```python
from build123d import *

# Parameters (mm, degrees)
SKETCH1_R           = 1.6
SKETCH1_R_2         = 2.5
BOSS_EXTRUDE1_DEPTH = 3


with BuildPart() as part:
    # Sketch1 → Boss-Extrude1 (new body)
    with BuildSketch(Plane.XY):
        with BuildLine():
            Line((168.027079905, 1038.043290918), (213.692404138, 1038.043292418))
            ThreePointArc((213.692404138, 1038.043292418), (215.106618088, 1038.62907792), (215.692405461, 1040.043291095))
            Line((215.692405461, 1040.043291095), (215.692425273, 1068.407217461))
            ThreePointArc((215.692425273, 1068.407217461), (215.037497189, 1069.988356706), (213.456358826, 1070.643286918))
            Line((213.456358826, 1070.643286918), (170.527157049, 1070.643286918))
            Line((170.527157049, 1070.643286918), (170.527154049, 1066.109317918))
            ThreePointArc((170.527154049, 1066.109317918), (170.594141198, 1065.85931758), (170.777154049, 1065.67630462))
            ThreePointArc((170.777154049, 1065.67630462), (170.880709235, 1064.889738733), (170.094142887, 1064.993290414))
            ThreePointArc((170.094142887, 1064.993290414), (169.911130301, 1065.176302052), (169.661131049, 1065.243288918))
            Line((169.661131049, 1065.243288918), (168.027102049, 1065.243288918))
            ThreePointArc((168.027102049, 1065.243288918), (167.673548658, 1065.096842309), (167.527102049, 1064.743288918))
            Line((167.527102049, 1064.743288918), (167.527102049, 1059.743291918))
            ThreePointArc((167.527102049, 1059.743291918), (167.673545881, 1059.389741498), (168.027094, 1059.243292111))
            Line((168.027094, 1059.243292111), (169.661121, 1059.243294985))
            ThreePointArc((169.661121, 1059.243294985), (169.911120776, 1059.310282365), (170.094133317, 1059.493294952))
            ThreePointArc((170.094133317, 1059.493294952), (170.880698604, 1059.596848318), (170.77714747, 1058.810282737))
            ThreePointArc((170.77714747, 1058.810282737), (170.594135891, 1058.627270291), (170.527148933, 1058.37727121))
            Line((170.527148933, 1058.37727121), (170.527145536, 1053.243292145))
            Line((170.527145536, 1053.243292145), (173.327145536, 1053.243292145))
            Line((173.327145536, 1053.243292145), (173.327146479, 1054.668300832))
            Line((173.327146479, 1054.668300832), (177.527142575, 1054.668300832))
            Line((177.527142575, 1054.668300832), (177.527142575, 1053.243290914))
            Line((177.527142575, 1053.243290914), (180.527142575, 1053.243292145))
            Line((180.527142575, 1053.243292145), (180.527142575, 1050.043292145))
            Line((180.527142575, 1050.043292145), (177.527142575, 1050.043292145))
            Line((177.527142575, 1050.043292145), (177.527142575, 1048.768300832))
            Line((177.527142575, 1048.768300832), (173.327142575, 1048.768300832))
            Line((173.327142575, 1048.768300832), (173.327143418, 1050.043292145))
            Line((173.327143418, 1050.043292145), (170.527143418, 1050.043292145))
            Line((170.527143418, 1050.043292145), (170.527140021, 1044.909316322))
            ThreePointArc((170.527140021, 1044.909316322), (170.594127154, 1044.659316277), (170.777139735, 1044.476303455))
            ThreePointArc((170.777139735, 1044.476303455), (170.8806944, 1043.689737499), (170.094128121, 1043.793289701))
            ThreePointArc((170.094128121, 1043.793289701), (169.911115656, 1043.97630146), (169.661116448, 1044.043288491))
            Line((169.661116448, 1044.043288491), (168.027087448, 1044.043289572))
            ThreePointArc((168.027087448, 1044.043289572), (167.673533961, 1043.896843197), (167.527087117, 1043.543289903))
            Line((167.527087117, 1043.543289903), (167.527083809, 1038.543292903))
            ThreePointArc((167.527083809, 1038.543292903), (167.673528336, 1038.189739609), (168.027079905, 1038.043290918))
        make_face()
        with Locations((195.192419253, 1056.643286172)):
            Circle(SKETCH1_R, mode=Mode.SUBTRACT)
        with Locations((205.192419253, 1056.643286172)):
            Circle(SKETCH1_R_2, mode=Mode.SUBTRACT)
    extrude(amount=BOSS_EXTRUDE1_DEPTH)


solid = part.part
```
Can you work these out from the model? Positions are in its coordinate system, mm. A direction names the side the tool comes from. Round coordinates to 2 decimals unless told otherwise and drop trailing zeros. Loops run counter-clockwise (first coordinate to the right, second up) from the corner with the lowest first, then second, coordinate; pieces in that order, holes last. Notation, with made-up numbers: M -4.75,33.5 L 10.25,33.5 A22 ccw 10.25,52.5 Z; hole C -27.75,28.25 d4. An arc over 180 degrees is marked long. Write item = value, one per line. Start each with the question number.
(1) Suppose I cut it at B-B on y = 1067. Write out the boundary of the cut face in (x, z).
(2) I need wall thicknesses on line 1 along X through (y, z) = (1058, 2.2); line 2 along Y through (x, z) = (175.5, 0.6); line 3 along X through (y, z) = (1050, 2.5). Which ranges of each line are inside material? Lowest first, please.
(3) Which directions (+Z, -Z, +X, -X, +Y, -Y) give clear straight access to the entire face, cutting with the end or side of a thin tool? Please do faces 1 (the face through (172, 1053.243, 1)), 2 (the face through (191, 1038.043, 1)), 3 (the face through (175, 1054.668, 1)).
(4) Suppose I cut it at D-D on x = 205.5. Write out the boundary of the cut face in (y, z), plus the area to 3 significant figures.
(5) Suppose I cut it at A-A on x = 176.5. Write out the boundary of the cut face in (y, z).
(6) Suppose I cut it at C-C on z = 1. Give the number of separate pieces and of enclosed holes in the cut face, plus the area to 3 significant figures.
(7) I'm going to push flat-ended pins straight in: P1, Ø1.5, axis at y = 1068, z = 1, coming from the -X side; P2, Ø1.2, axis at x = 170.53, y = 1065.24, coming from the -Z side. Where does each tip first touch, or does it pass through?
(8) If we mould it in two halves opening along X, with no side actions, what happens to faces 4 (the face through (170.527, 1068, 1)), 5 (the face through (177.527, 1049, 1)), 6 (the face through (191, 1055, 0))? For each: released by +X, released by -X, zero draft, split by the parting line, or undercut.
Answer block:
q1.outline = M 170.53,0 L 215.69,0 L 215.69,3 L 170.53,3 Z
q2.line_1 = 170.53 to 194.34, 196.04 to 203.09, 207.29 to 215.69
q2.line_2 = 1038.04 to 1048.77, 1054.67 to 1070.64
q2.line_3 = 170.53 to 173.33, 177.53 to 215.69
q3.face_1 = +Z, -Z, -X
q3.face_2 = +Z, -Z, +X, -X, -Y
q3.face_3 = +Z, -Z
q4.outline = M 1038.04,0 L 1054.16,0 L 1054.16,3 L 1038.04,3 Z; M 1059.12,0 L 1070.64,0 L 1070.64,3 L 1059.12,3 Z
q4.area = 82.9 mm²
q5.outline = M 1038.04,0 L 1048.77,0 L 1048.77,3 L 1038.04,3 Z; M 1054.67,0 L 1070.64,0 L 1070.64,3 L 1054.67,3 Z
q6.separate_pieces = 1
q6.enclosed_holes = 2
q6.area = 1,430 mm²
q7.P1 = 170.53
q7.P2 = 0
q8.face_4 = released by -X
q8.face_5 = undercut
q8.face_6 = zero draft
